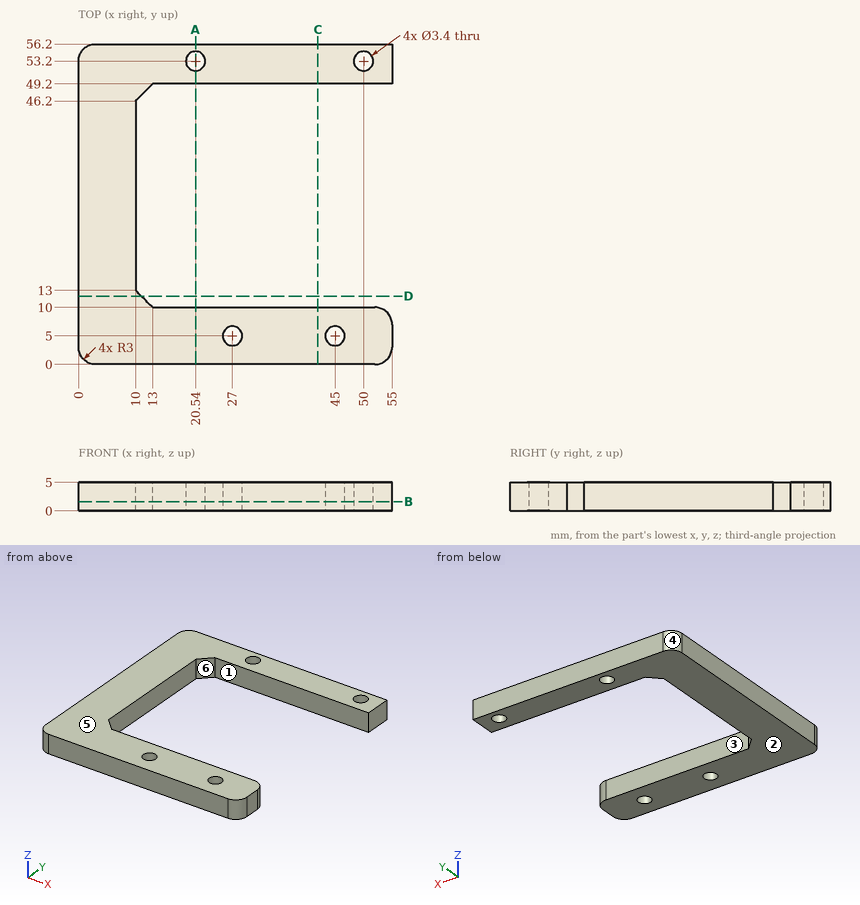
Design review of the part shown in the three views and the two pictorial views. Dimensions are in mm from the part's minimum x, y and z. A direction names the side the tool comes from. Round coordinates to 2 decimals unless told otherwise and drop trailing zeros. Write each loop counter-clockwise with the first axis right and the second up, starting at its lowest first coordinate (ties: lowest second). Pieces come first, ordered by that corner, then holes. Notation, with made-up numbers: (8.5, 29) -> (27.5, 29) arc R22 ccw to (27.5, 62) -> close; hole circle Ø5 at (81, 17). An arc over 180 degrees is marked (long way). Write item = value, one per line. Start each with the question number.
1) Tool access review of the marked faces 5 and 6: name each direction out of +Z, -Z, +X, -X, +Y, -Y from which nothing blocks a thin tool from reaching the whole face with its end or side.
2) Take a section at D-D, the plane y = 12. State the section outline as (x, z) points, plus the area to 3 significant figures.
3) Wall thickness on probe 1 along Y at (x, z) = (20.54, 1); probe 2 along Y at (x, z) = (27, 1.35); probe 3 along Y at (x, z) = (16, 4.5): over which ranges is each line inside the solid? List them lowest first. Write a range as from..to.
4) Mouldability with a two-part tool opening along Y and no side actions: class the marked faces 1, 2, 3 and 4 as +Y half, -Y half, draft (parallel to the pull), parting line (faces both ways), or undercut.
5) Take a section at A-A, the plane x = 20.54. State the section outline as (y, z) points, plus the area to 3 significant figures.
6) Clearance check with flat-ended pins moving along their axes: pin 1 (8 mm diameter, centred on x = 10, y = 49.5, fed in from -Z); pin 2 (1.5 mm diameter, centred on y = 22, z = 2.5, fed in from +X). State where each tip first meets the part, or that it passes through.
7) Take a section at B-B, the plane z = 1.65. State the section outline as (x, y) points, plus the area to 3 significant figures.
8) Take a section at C-C, the plane x = 42. State the section outline as (y, z) points.
Results list:
q1.face_5 = +Z, +X, -X, +Y, -Y
q1.face_6 = +Z, -Z, +X
q2.outline = (0, 0) -> (11, 0) -> (11, 5) -> (0, 5) -> close
q2.area = 55.0 mm²
q3.probe_1 = 0..10, 49.2..51.5, 54.9..56.2
q3.probe_2 = 0..3.3, 6.7..10, 49.2..56.2
q3.probe_3 = 0..10, 49.2..56.2
q4.face_1 = undercut
q4.face_2 = draft
q4.face_3 = undercut
q4.face_4 = +Y half
q5.outline = (0, 0) -> (10, 0) -> (10, 5) -> (0, 5) -> close; (49.2, 0) -> (51.5, 0) -> (51.5, 5) -> (49.2, 5) -> close; (54.9, 0) -> (56.2, 0) -> (56.2, 5) -> (54.9, 5) -> close
q5.area = 68.0 mm²
q6.pin_1 = 0
q6.pin_2 = 10
q7.outline = (0, 3) arc R3 ccw to (3, 0) -> (52, 0) arc R3 ccw to (55, 3) -> (55, 7) arc R3 ccw to (52, 10) -> (13, 10) -> (10, 13) -> (10, 46.2) -> (13, 49.2) -> (55, 49.2) -> (55, 56.2) -> (3, 56.2) arc R3 ccw to (0, 53.2) -> close; hole circle Ø3.4 at (20.54, 53.2); hole circle Ø3.4 at (27, 5); hole circle Ø3.4 at (45, 5); hole circle Ø3.4 at (50, 53.2)
q7.area = 1,290 mm²
q8.outline = (0, 0) -> (10, 0) -> (10, 5) -> (0, 5) -> close; (49.2, 0) -> (56.2, 0) -> (56.2, 5) -> (49.2, 5) -> close
